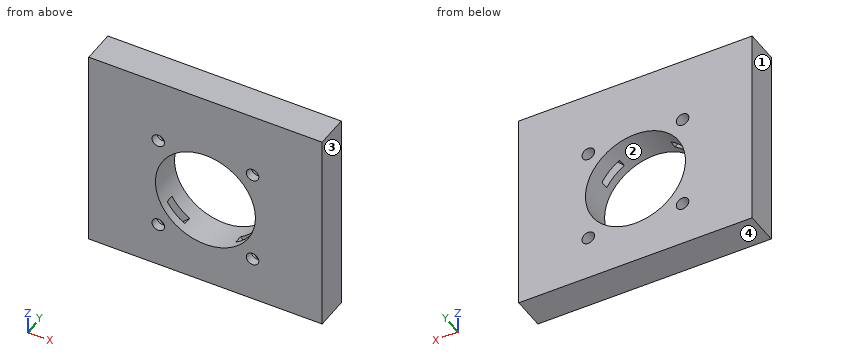
```python
from build123d import *

# Parameters (mm, degrees)
BOX786_W                    = 6
BOX786_H                    = 2
BOX786_DEPTH                = 8
BOX780_W                    = 8
BOX780_H                    = 2
BOX780_DEPTH                = 6
BOX783_W                    = 8
BOX783_H                    = 2
BOX783_DEPTH                = 6
BOX785_W                    = 6
BOX785_H                    = 2
BOX785_DEPTH                = 8
COMPOUND939_PLACEMENT_ANGLE = 45
CYLINDER1872_R              = 12
CYLINDER1872_DEPTH          = 20
CYLINDER1874_R              = 1.5
CYLINDER1874_DEPTH          = 40
CYLINDER1876_R              = 1.5
CYLINDER1876_DEPTH          = 40
CYLINDER1875_R              = 1.5
CYLINDER1875_DEPTH          = 40
CYLINDER1873_R              = 1.5
CYLINDER1873_DEPTH          = 40
COMPOUND942_PLACEMENT_ANGLE = 45
BOX782_W                    = 56
BOX782_H                    = 8
BOX782_DEPTH                = 49


with BuildPart() as krychle786:
    # Box786 → Box786 (new body)
    with BuildSketch(Plane(origin=(-3, 116, 30), x_dir=(1, 0, 0), z_dir=(0, 0, 1))):
        with Locations((3, 1)):
            Rectangle(BOX786_W, BOX786_H)
    extrude(amount=BOX786_DEPTH)


with BuildPart() as krychle780:
    # Box780 → Box780 (new body)
    with BuildSketch(Plane(origin=(-19, 116, 46), x_dir=(1, 0, 0), z_dir=(0, 0, 1))):
        with Locations((4, 1)):
            Rectangle(BOX780_W, BOX780_H)
    extrude(amount=BOX780_DEPTH)


with BuildPart() as krychle783:
    # Box783 → Box783 (new body)
    with BuildSketch(Plane(origin=(11, 116, 46), x_dir=(1, 0, 0), z_dir=(0, 0, 1))):
        with Locations((4, 1)):
            Rectangle(BOX783_W, BOX783_H)
    extrude(amount=BOX783_DEPTH)


with BuildPart() as compound939:
    # Box785 → Box785 (new body)
    with BuildSketch(Plane(origin=(-3, 116, 60), x_dir=(1, 0, 0), z_dir=(0, 0, 1))):
        with Locations((3, 1)):
            Rectangle(BOX785_W, BOX785_H)
    extrude(amount=BOX785_DEPTH)

    # Compound939: union Krychle786, Krychle780, Krychle783
    add(krychle786.part)
    add(krychle780.part)
    add(krychle783.part)


with BuildPart() as compound939_1:
    # Compound939 placement: moved
    add(compound939.part.moved(Location((-34.65, 0, 16.35))).rotate(Axis((-34.65, 0, 16.35), (0, 1, 0)), COMPOUND939_PLACEMENT_ANGLE))


with BuildPart() as obj1:
    # Cylinder1872 → Cylinder1872 (new body)
    with BuildSketch(Plane(origin=(0, 124, 51), x_dir=(1, 0, 0), z_dir=(0, -1, 0))):
        Circle(CYLINDER1872_R)
    extrude(amount=CYLINDER1872_DEPTH)


with BuildPart() as obj2:
    # Cylinder1874 → Cylinder1874 (new body)
    with BuildSketch(Plane(origin=(16, 140, 49), x_dir=(1, 0, 0), z_dir=(0, -1, 0))):
        Circle(CYLINDER1874_R)
    extrude(amount=CYLINDER1874_DEPTH)


with BuildPart() as obj3:
    # Cylinder1876 → Cylinder1876 (new body)
    with BuildSketch(Plane(origin=(-16, 140, 49), x_dir=(1, 0, 0), z_dir=(0, -1, 0))):
        Circle(CYLINDER1876_R)
    extrude(amount=CYLINDER1876_DEPTH)


with BuildPart() as obj4:
    # Cylinder1875 → Cylinder1875 (new body)
    with BuildSketch(Plane(origin=(0, 140, 33), x_dir=(1, 0, 0), z_dir=(0, -1, 0))):
        Circle(CYLINDER1875_R)
    extrude(amount=CYLINDER1875_DEPTH)


with BuildPart() as compound942:
    # Cylinder1873 → Cylinder1873 (new body)
    with BuildSketch(Plane(origin=(0, 140, 65), x_dir=(1, 0, 0), z_dir=(0, -1, 0))):
        Circle(CYLINDER1873_R)
    extrude(amount=CYLINDER1873_DEPTH)

    # Compound942: union obj2, obj3, obj4
    add(obj2.part)
    add(obj3.part)
    add(obj4.part)


with BuildPart() as compound942_1:
    # Compound942 placement: moved
    add(compound942.part.moved(Location((-34.65, 0, 16.35))).rotate(Axis((-34.65, 0, 16.35), (0, 1, 0)), COMPOUND942_PLACEMENT_ANGLE))


with BuildPart() as cut588:
    # Box782 → Box782 (new body)
    with BuildSketch(Plane(origin=(-28, 114, 29), x_dir=(1, 0, 0), z_dir=(0, 0, 1))):
        with Locations((28, 4)):
            Rectangle(BOX782_W, BOX782_H)
    extrude(amount=BOX782_DEPTH)

    # Cut584: cut Compound942
    add(compound942_1.part, mode=Mode.SUBTRACT)

    # Cut590: cut obj1
    add(obj1.part, mode=Mode.SUBTRACT)

    # Cut588: cut Compound939
    add(compound939_1.part, mode=Mode.SUBTRACT)


solid = cut588.part
```
Design review of the part built by this model. Coordinates are the model's own, in mm. Face numbers are marked on the shaded views. Round coordinates to 2 decimals unless told otherwise and drop trailing zeros. Write each loop counter-clockwise with the first axis right and the second up, starting at its lowest first coordinate (ties: lowest second). Pieces come first, ordered by that corner, then holes.
Item 1: We need section C-C on y = 121. Write out the cut boundary in (x, z).
Item 2: We need section A-A on x = 0. Write out the cut boundary in (y, z).
Item 3: For probe 1 along Y at (x, z) = (10.5, 61); probe 2 along Z at (x, y) = (0, 118.5); probe 3 along X at (y, z) = (118.25, 61.5), list the stretches that pass through material, from the lowest coordinate up.
Item 4: The part is to be moulded in two halves that separate along X. For the marked faces 1, 2, 3 and 4, say which applies: +X half, -X half, draft (parallel to the pull), parting line (faces both ways), or undercut.
Item 5: We need section B-B on z = 51. Write out the cut boundary in (x, y).
Item 6: We need section D-D on x = -7. Write out the cut boundary in (y, z).
Item 7: Clearance check with a flat-ended pin moving along its axis: pin 1 Ø3.5 at (x, z) = (11.31, 39.68) entering from -Y. State where the tip first meets the part, or that it passes through.
Returned:
1. outline: (-28, 29) - (28, 29) - (28, 78) - (-28, 78) - close; hole circle Ø3 at (-11.32, 39.68); hole circle Ø3 at (-11.32, 62.31); hole circle Ø24 at (0, 51); hole circle Ø3 at (11.31, 39.68); hole circle Ø3 at (11.31, 62.31)
2. outline: (114, 29) - (122, 29) - (122, 39) - (114, 39) - close; (114, 63) - (122, 63) - (122, 78) - (114, 78) - close
3. probe 1: y = 114 to 116, 118 to 122
3. probe 2: z = 29 to 39, 63 to 78
3. probe 3: x = -28 to -12.58, -10.05 to -5.81, 5.81 to 10.05, 12.57 to 28
4. face 1: -X half
4. face 2: undercut
4. face 3: +X half
4. face 4: draft
5. outline: (-28, 114) - (-12, 114) - (-12, 122) - (-28, 122) - close; (12, 114) - (28, 114) - (28, 122) - (12, 122) - close
6. outline: (114, 29) - (122, 29) - (122, 41.25) - (118, 41.25) - (118, 39.76) - (116, 39.76) - (116, 41.25) - (114, 41.25) - close; (114, 60.75) - (116, 60.75) - (116, 62.24) - (118, 62.24) - (118, 60.75) - (122, 60.75) - (122, 78) - (114, 78) - close
7. pin 1: stops at y = 114
